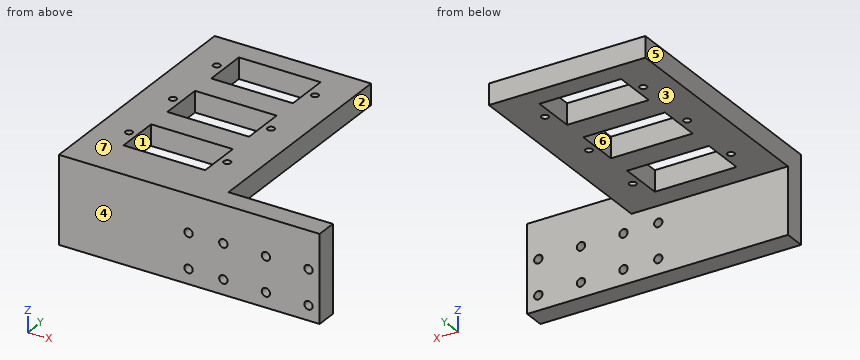
```python
from build123d import *

# Parameters (mm, degrees)
SKETCH1_W           = 45
SKETCH1_H           = 6
BOSS_EXTRUDE1_DEPTH = 65
SKETCH2_R           = 1
SKETCH2_W           = 23.5
SKETCH2_H           = 12.6
CUT_EXTRUDE1_DEPTH  = 80.284298572
LPATTERN1_COUNT     = 3
LPATTERN1_PITCH     = 20
SKETCH3_W           = 45
SKETCH3_H           = 25
BOSS_EXTRUDE2_DEPTH = 6
SKETCH4_W           = 25
SKETCH4_H           = 6
BOSS_EXTRUDE3_DEPTH = 30
SKETCH5_R           = 1.2
CUT_EXTRUDE2_DEPTH  = 107.259117256


with BuildPart() as part:
    # Sketch1 → Boss-Extrude1 (new body)
    with BuildSketch(Plane(origin=(0, 0, 0), x_dir=(1, 0, 0), z_dir=(0, 1, 0))):
        with Locations((22.5, 3)):
            Rectangle(SKETCH1_W, SKETCH1_H)
    extrude(amount=BOSS_EXTRUDE1_DEPTH)

    # Sketch2 → Cut-Extrude1 (cut, through all)
    with BuildSketch(Plane.XY):
        with Locations((8.375, 52.7)):
            Circle(SKETCH2_R)
        with Locations((36.625, 52.7)):
            Circle(SKETCH2_R)
        with Locations((22.5, 52.7)):
            Rectangle(SKETCH2_W, SKETCH2_H)
    cut_extrude1 = extrude(amount=-CUT_EXTRUDE1_DEPTH, mode=Mode.SUBTRACT)

    # LPattern1: Cut-Extrude1 ×3
    with Locations(*[(0, -i * LPATTERN1_PITCH, 0) for i in range(1, LPATTERN1_COUNT)]):
        add(cut_extrude1, mode=Mode.SUBTRACT)

    # Sketch3 → Boss-Extrude2 (add)
    with BuildSketch(Plane.XZ):
        with Locations((22.5, -12.5)):
            Rectangle(SKETCH3_W, SKETCH3_H)
    extrude(amount=BOSS_EXTRUDE2_DEPTH)

    # Sketch4 → Boss-Extrude3 (add)
    with BuildSketch(Plane(origin=(45, 0, 0), x_dir=(0, 0, -1), z_dir=(1, 0, 0))):
        with Locations((12.5, -3)):
            Rectangle(SKETCH4_W, SKETCH4_H)
    extrude(amount=BOSS_EXTRUDE3_DEPTH)

    # Sketch5 → Cut-Extrude2 (cut, through all)
    with BuildSketch(Plane.XZ.offset(6)):
        with Locations(Location((37.288839919, -20.74934001, 0), (0, 0, 270))):
            Circle(SKETCH5_R)
        with Locations(Location((37.288839919, -10.74934001, 0), (0, 0, 270))):
            Circle(SKETCH5_R)
        with Locations(Location((47.288839919, -20.74934001, 0), (0, 0, 270))):
            Circle(SKETCH5_R)
        with Locations(Location((47.288839919, -10.74934001, 0), (0, 0, 270))):
            Circle(SKETCH5_R)
        with Locations(Location((59.538839919, -20.74934001, 0), (0, 0, 270))):
            Circle(SKETCH5_R)
        with Locations(Location((71.788839919, -20.74934001, 0), (0, 0, 270))):
            Circle(SKETCH5_R)
        with Locations(Location((71.788839919, -10.74934001, 0), (0, 0, 270))):
            Circle(SKETCH5_R)
        with Locations(Location((59.538839919, -10.74934001, 0), (0, 0, 270))):
            Circle(SKETCH5_R)
    extrude(amount=-CUT_EXTRUDE2_DEPTH, mode=Mode.SUBTRACT)


solid = part.part
```
Part model, mm, in its own coordinate system. Face numbers are marked on the shaded views. A direction names the side the tool comes from. Coordinates: 2 decimals unless noted, no trailing zeros. Write each loop counter-clockwise with the first axis right and the second up, starting at its lowest first coordinate (ties: lowest second). Pieces come first, ordered by that corner, then holes.
Item 1: Slice it at B-B (x = 31.5). Write the cut outline in (y, z), and give its area (3 significant figures).
Item 2: Slice it at C-C (z = -4.5). Count the separate pieces of the cut face and the enclosed holes in it, and give its area (3 significant figures).
Item 3: Pin check, flat tips, straight feed: pin 1 (3 mm diameter, centred on x = 37.29, z = -10.75, fed in from +Y); pin 2 (1.2 mm diameter, centred on x = 36.625, y = 52.7, fed in from -Z); pin 3 (2.5 mm diameter, centred on x = 8.375, y = 32.7, fed in from -Z); pin 4 (6.5 mm diameter, centred on y = 13, z = -3, fed in from +X). Stop position of each tip, or through.
Item 4: Slice it at A-A (y = 36.5). Write the cut outline in (x, z).
Item 5: Slice it at D-D (x = 41). Write the cut outline in (y, z), and give its area (3 significant figures).
Item 6: Mould opens along X. For the marked faces 5, 6 and 7 say: released by +X, released by -X, zero draft, split by the parting line, or undercut.
Item 7: Probe line 1 (X direction, y = 11, z = -2.5); line 2 (Y direction, x = 61, z = -23). List the from-to ranges inside material, lowest first.
Item 8: Which spindle directions (+Z, -Z, +X, -X, +Y, -Y) get a long thin tool onto all of the face, cutting with end or side? Do the marked faces 1, 2, 3 and 4. Say none if no direction does.
Results found:
1. outline: (-6, -25) - (0, -25) - (0, -6) - (6.4, -6) - (6.4, 0) - (-6, 0) - close; (19, -6) - (26.4, -6) - (26.4, 0) - (19, 0) - close; (39, -6) - (46.4, -6) - (46.4, 0) - (39, 0) - close; (59, -6) - (65, -6) - (65, 0) - (59, 0) - close
1. area: 313 mm2
2. separate pieces: 1
2. enclosed holes: 9
2. area: 2,470 mm2
3. pin 1: stops at y = 0
3. pin 2: passes through
3. pin 3: stops at z = -6
3. pin 4: stops at x = 45
4. outline: (0, -6) - (10.75, -6) - (10.75, 0) - (0, 0) - close; (34.25, -6) - (45, -6) - (45, 0) - (34.25, 0) - close
5. outline: (-6, -25) - (0, -25) - (0, -6) - (65, -6) - (65, 0) - (-6, 0) - close
5. area: 540 mm2
6. face 5: released by -X
6. face 6: undercut
6. face 7: zero draft
7. line 1: x = 0 to 10.75, 34.25 to 45
7. line 2: y = -6 to 0
8. face 1: +Z, -Z
8. face 2: +Z, -Z, +X, +Y
8. face 3: -Z, +X, -X, +Y
8. face 4: +Z, -Z, +X, -X, -Y
